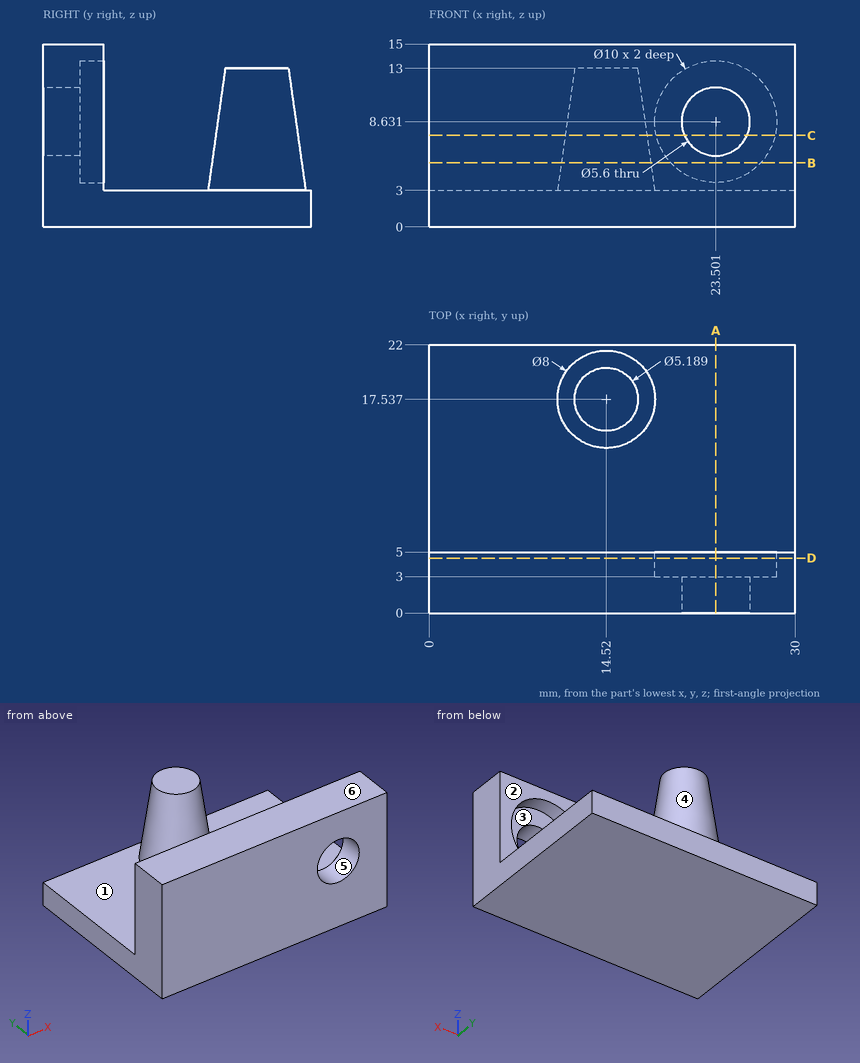
Geometry: see drawing. Coordinates: mm, zero at the bounding-box minimum. A direction names the side the tool comes from. Give positions to 0.01 mm unless a question says otherwise; leave off trailing zeros. Loops run counter-clockwise (first coordinate to the right, second up) from the corner with the lowest first, then second, coordinate; pieces in that order, holes last. Notation, with made-up numbers: (-18.75, 76) -> (26.25, 76) arc R35 ccw to (26.25, 109) -> close; hole circle Ø11 at (66, 63). An arc over 180 degrees is marked (long way). Answer as a JSON object with one key per item and string values. Group by question number.
Item 1: Reachability of the marked faces 1, 2 and 3 from +Z, -Z, +X, -X, +Y, -Y: full face, straight path, thin tool, end or side. Return the list, or none.
Item 2: Cut plane D-D, the plane y = 4.5. Return the cut outline in (x, z).
Item 3: Pull-direction query (X, two-part tool) for the marked faces 4, 5 and 6; classes: released by +X, released by -X, zero draft, split by the parting line, or undercut.
Item 4: Line query: probe 1 along Z at (x, y) = (5, 12.75); probe 2 along Y at (x, z) = (4, 9.25); probe 3 along Y at (x, z) = (14.5, 10). Output: solid intervals per line, ascending.
Item 5: Cut plane C-C, the plane z = 7.5. Return the cut outline in (x, y) (1 decimal), and give its area (3 significant figures).
Item 6: Cut plane A-A, the plane x = 23.5. Return the cut outline in (y, z).
Item 7: Cut plane B-B, the plane z = 5.25. Return the cut outline in (x, y) (1 decimal).
Item 8: Pin query (flat end, axial travel): P1, Ø6.5, axis at x = 23.5, z = 8.63, coming from the +Y side; P2, Ø2.5, axis at x = 15.5, y = 16.5, coming from the +Z side; P3, Ø6, axis at x = 17, z = 9.5, coming from the +Y side. Return the tip coordinate at first contact, or that it passes through.
Checks:
{
 "1": {"face 1": "+Z", "face 2": "+Z, +X, -X", "face 3": "+Y"},
 "2": {"outline": "(0, 0) -> (30, 0) -> (30, 15) -> (0, 15) -> close; hole circle Ø10 at (23.5, 8.63)"},
 "3": {"face 4": "split by the parting line", "face 5": "undercut", "face 6": "zero draft"},
 "4": {"probe 1": "z = 0 to 3", "probe 2": "y = 0 to 5", "probe 3": "y = 0 to 5, 14.52 to 20.55"},
 "5": {"outline": "(0, 0) -> (20.9, 0) -> (20.9, 3) -> (18.6, 3) -> (18.6, 5) -> (0, 5) -> close; circle Ø6.7 at (14.5, 17.5); (26.1, 0) -> (30, 0) -> (30, 5) -> (28.4, 5) -> (28.4, 3) -> (26.1, 3) -> close", "area": "151 mm²"},
 "6": {"outline": "(0, 0) -> (22, 0) -> (22, 3) -> (5, 3) -> (5, 3.63) -> (3, 3.63) -> (3, 5.83) -> (0, 5.83) -> close; (0, 11.43) -> (3, 11.43) -> (3, 13.63) -> (5, 13.63) -> (5, 15) -> (0, 15) -> close"},
 "7": {"outline": "(0, 0) -> (30, 0) -> (30, 5) -> (27.2, 5) -> (27.2, 3) -> (19.8, 3) -> (19.8, 5) -> (0, 5) -> close; circle Ø7.4 at (14.5, 17.5)"},
 "8": {"P1": "stops at y = 3", "P2": "stops at z = 13", "P3": "stops at y = 20.9"}
}
